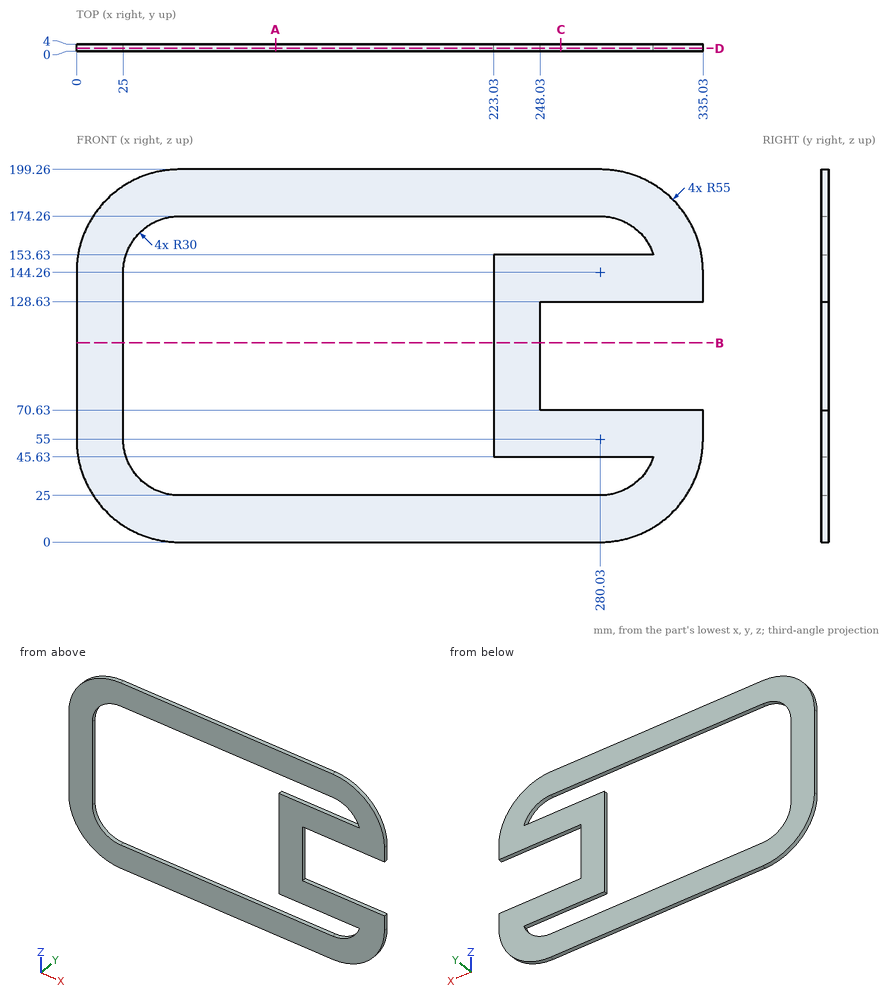
The figure shows three views and two pictorial views of one solid part (mm, origin at its lowest corner). Answer the questions. Round coordinates to 2 decimals unless told otherwise and drop trailing zeros. Loops run counter-clockwise (first coordinate to the right, second up) from the corner with the lowest first, then second, coordinate; pieces in that order, holes last. Notation, with made-up numbers: (8.25, 24) - (27.25, 24) arc R17 cw to (27.25, 42) - close; hole circle Ø2 at (54.25, -30). An arc over 180 degrees is marked (long way). One line per question, with ' | ' between items. Start each with the question number.
Q1. Section C-C on x = 259 is taken. Give the vertices of the cut face in (y, z).
Q2. Section D-D on y = 1.7 is taken. Give the vertices of the cut face in (x, z).
Q3. Find the intervals of material crossed by L1, parallel to Z at x = 256, y = 0.6; L2, parallel to Z at x = 85.5, y = 1.8; L3, parallel to X at y = 3.75, z = 110, in increasing order.
Q4. Flat-ended cylindrical pins translate along their axes: pin 1 (2 mm diameter, centred on x = 305.5, y = 1.5, fed in from -Z); pin 2 (1.2 mm diameter, centred on x = 281.5, y = 2.5, fed in from -Z). Find the tip coordinate at first contact, or state that the pin passes through.
Q5. Section B-B on z = 106.5 is taken. Give the vertices of the cut face in (x, y), plus the area to 3 significant figures.
Q6. Section A-A on x = 106.5 is taken. Give the vertices of the cut face in (y, z), plus the area to 3 significant figures.
Established:
1) outline: (0, 0) - (4, 0) - (4, 25) - (0, 25) - close; (0, 45.63) - (4, 45.63) - (4, 70.63) - (0, 70.63) - close; (0, 128.63) - (4, 128.63) - (4, 153.63) - (0, 153.63) - close; (0, 174.26) - (4, 174.26) - (4, 199.26) - (0, 199.26) - close
2) outline: (0, 55) arc R55 ccw to (55, 0) - (280.03, 0) arc R55 ccw to (335.03, 55) - (335.03, 70.63) - (248.03, 70.63) - (248.03, 128.63) - (335.03, 128.63) - (335.03, 144.26) arc R55 ccw to (280.03, 199.26) - (55, 199.26) arc R55 ccw to (0, 144.26) - close; hole (25, 55) arc R30 ccw to (55, 25) - (280.03, 25) arc R30 ccw to (308.53, 45.63) - (223.03, 45.63) - (223.03, 153.63) - (308.53, 153.63) arc R30 ccw to (280.03, 174.26) - (55, 174.26) arc R30 ccw to (25, 144.26) - close
3) L1: 0 to 25, 45.63 to 70.63, 128.63 to 153.63, 174.26 to 199.26 | L2: 0 to 25, 174.26 to 199.26 | L3: 0 to 25, 223.03 to 248.03
4) pin 1: z = 5.74 | pin 2: z = 0.01
5) outline: (0, 0) - (25, 0) - (25, 4) - (0, 4) - close; (223.03, 0) - (248.03, 0) - (248.03, 4) - (223.03, 4) - close | area: 200 mm²
6) outline: (0, 0) - (4, 0) - (4, 25) - (0, 25) - close; (0, 174.26) - (4, 174.26) - (4, 199.26) - (0, 199.26) - close | area: 200 mm²
